```python
from build123d import *

# Parameters (mm, degrees)
SKETCH1_W           = 69
SKETCH1_H           = 46
BOSS_EXTRUDE1_DEPTH = 10
SKETCH2_R           = 19
SKETCH2_R_2         = 9
BOSS_EXTRUDE2_DEPTH = 25
BOSS_EXTRUDE3_DEPTH = 19
FILLET1_R           = 30
FILLET2_R           = 10
RIB1_START          = -5
RIB1_DEPTH          = 10
FILLET3_R           = 25
SKETCH7_R           = 8
CUT_EXTRUDE1_DEPTH  = 38


# Read off the part's stored shape, not the designer's step: Rib1
with BuildPart() as part:
    # Sketch1 → Boss-Extrude1 (new body)
    with BuildSketch(Plane(origin=(0, 0, 0), x_dir=(0, 1, 0), z_dir=(0, 0, 1))):
        Rectangle(SKETCH1_W, SKETCH1_H)
    extrude(amount=BOSS_EXTRUDE1_DEPTH)



with BuildPart() as body_2:
    # Sketch2 → Boss-Extrude2 (new body)
    with BuildSketch(Plane(origin=(0, 0, 113), x_dir=(-1, 0, 0), z_dir=(0, 0, -1))):
        with Locations((52, -15.5)):
            Circle(SKETCH2_R)
        with Locations((52, -15.5)):
            Circle(SKETCH2_R_2, mode=Mode.SUBTRACT)
    extrude(amount=BOSS_EXTRUDE2_DEPTH)


with BuildPart() as part_1:
    add(part.part)

    add(body_2.part)  # Boss-Extrude3 merges body 2
    # Sketch5 → Boss-Extrude3 (add, symmetric)
    with BuildSketch(Plane(origin=(0, -15.5, 0), x_dir=(-1, 0, 0), z_dir=(0, -1, 0))):
        Polygon((23, -10), (23, -90.5), (52.274133124, -90.5), (52.274133124, -100.5), (13, -100.5), (13, -10), align=None)
    extrude(amount=BOSS_EXTRUDE3_DEPTH, both=True)

    # Fillet1
    fillet1_edges = [part_1.edges().sort_by_distance(p)[0] for p in [
        (-18, 3.5, 10),
    ]]
    fillet(fillet1_edges, radius=FILLET1_R)

    # Fillet2
    fillet2_edges = [part_1.edges().sort_by_distance(p)[0] for p in [
        (-23, -15.5, 90.5),
    ]]
    fillet(fillet2_edges, radius=FILLET2_R - 0.0001)  # a hair under: the kernel refuses the full size
    fillet2_2_edges = [part_1.edges().sort_by_distance(p)[0] for p in [
        (-13, -15.5, 100.5),
    ]]
    fillet(fillet2_2_edges, radius=FILLET2_R)

    # Rib1 outline → Rib1 (add)
    with BuildSketch(Plane(origin=(0, -15.5, 0), x_dir=(-1, 0, 0), z_dir=(0, -1, 0)).offset(RIB1_START)):
        with BuildLine():
            Line((23, -110.5), (35, -110.5))
            Line((35, -110.5), (35, -100.5))
            Line((35, -100.5), (23, -100.5))
            ThreePointArc((23, -100.5), (15.928932188, -97.571067812), (13, -90.5))
            Line((13, -90.5), (13, -10))
            Line((13, -10), (3, -10))
            Line((3, -10), (3, -90.5))
            ThreePointArc((3, -90.5), (8.857864376, -104.642135624), (23, -110.5))
        make_face()
    extrude(amount=RIB1_DEPTH)

    # Fillet3
    fillet3_edges = [part_1.edges().sort_by_distance(p)[0] for p in [
        (-3, -15.5, 10),
    ]]
    fillet(fillet3_edges, radius=FILLET3_R)

    # Sketch7 → Cut-Extrude1 (cut)
    with BuildSketch(Plane.XY.offset(10)):
        with Locations((5, 12.5)):
            Circle(SKETCH7_R)
    extrude(amount=-CUT_EXTRUDE1_DEPTH, mode=Mode.SUBTRACT)


solid = part_1.part
```
For this review, take the finished solid that the model builds, in its own axes (mm). A direction names the side the tool comes from. Round coordinates to 2 decimals unless told otherwise and drop trailing zeros. Write each loop counter-clockwise with the first axis right and the second up, starting at its lowest first coordinate (ties: lowest second). Pieces come first, ordered by that corner, then holes. Notation, with made-up numbers: (37.5, 89.5) - (54.5, 89.5) arc R23 ccw to (54.5, 121.5) - close; hole circle Ø6 at (38, 82). An arc over 180 degrees is marked (long way). Write each question's results on one line, items separated by ' | '.
Item 1: For faces 1 (the face through (-31, -2, 100.5)), 2 (the face through (-31, -29, 100.5)), 3 (the face through (-3, -15, 62)), 4 (the face through (-22.5, 3.5, 79.1)), list the 3-axis set-ups (+Z, -Z, +X, -X, +Y, -Y) from which the entire face can be reached by the end or side of a thin tool; tool diameter is ignored.
Calculated:
face 1: +Z, +X, +Y | face 2: +Z, +X, -Y | face 3: +Z, +X, +Y, -Y | face 4: +Z, +X, -X, +Y
Item 2: Take a section at C-C on x = 5. State the section outline as (y, z) points.
Calculated:
outline: (-34.5, 0) - (4.5, 0) - (4.5, 10) - (-10.5, 10) - (-10.5, 16.67) - (-20.5, 16.67) - (-20.5, 10) - (-34.5, 10) - close; (20.5, 0) - (34.5, 0) - (34.5, 10) - (20.5, 10) - close
Item 3: Draft analysis for pull direction Y (two halves, no side actions). For faces 5 (the face through (0, 34.5, 5)), 6 (the face through (-15.85, -27.6, 97.49)), 7 (the face through (-18, -34.5, 50)), 8 (the face through (8.69, 5.4, 5.07)), state which applies: pulls with the +Y half, pulls with the -Y half, needs draft (parallel to the pull), parting line crosses it, or undercut.
Calculated:
face 5: pulls with the +Y half | face 6: needs draft | face 7: pulls with the -Y half | face 8: undercut
Item 4: For pin 1 (10 mm diameter, centred on x = -46.5, y = -18.5, fed in from +Z); pin 2 (4.5 mm diameter, centred on x = -48, y = -19, fed in from -Z); pin 3 (1.5 mm diameter, centred on x = -23, z = 35, fed in from +Y); pin 4 (5 mm diameter, centred on y = -12, z = 82.5, fed in from -X), all flat-tipped, find the tip position at first contact; note any pin that passes through.
Calculated:
pin 1: stops at z = 113 | pin 2: stops at z = 90.5 | pin 3: stops at y = 4.06 | pin 4: stops at x = -24.07
Item 5: Take a section at B-B on z = 77.5. State the section outline as (x, y) points.
Calculated:
outline: (-23, -34.5) - (-13, -34.5) - (-13, -20.5) - (-3, -20.5) - (-3, -10.5) - (-13, -10.5) - (-13, 3.5) - (-23, 3.5) - close
Item 6: To check wall thickness, follow line 1 along Y through (x, z) = (5, 4.5); line 2 along X through (y, z) = (12, 5); line 3 along Y through (x, z) = (-52, 101.5). State the ranges of each line that lie inside material, in increasing order. Write a range as from..to.
Calculated:
line 1: y = -34.5..4.5, 20.5..34.5 | line 2: x = -23..-2.98, 12.98..23 | line 3: y = -34.5..-24.5, -6.5..3.5
